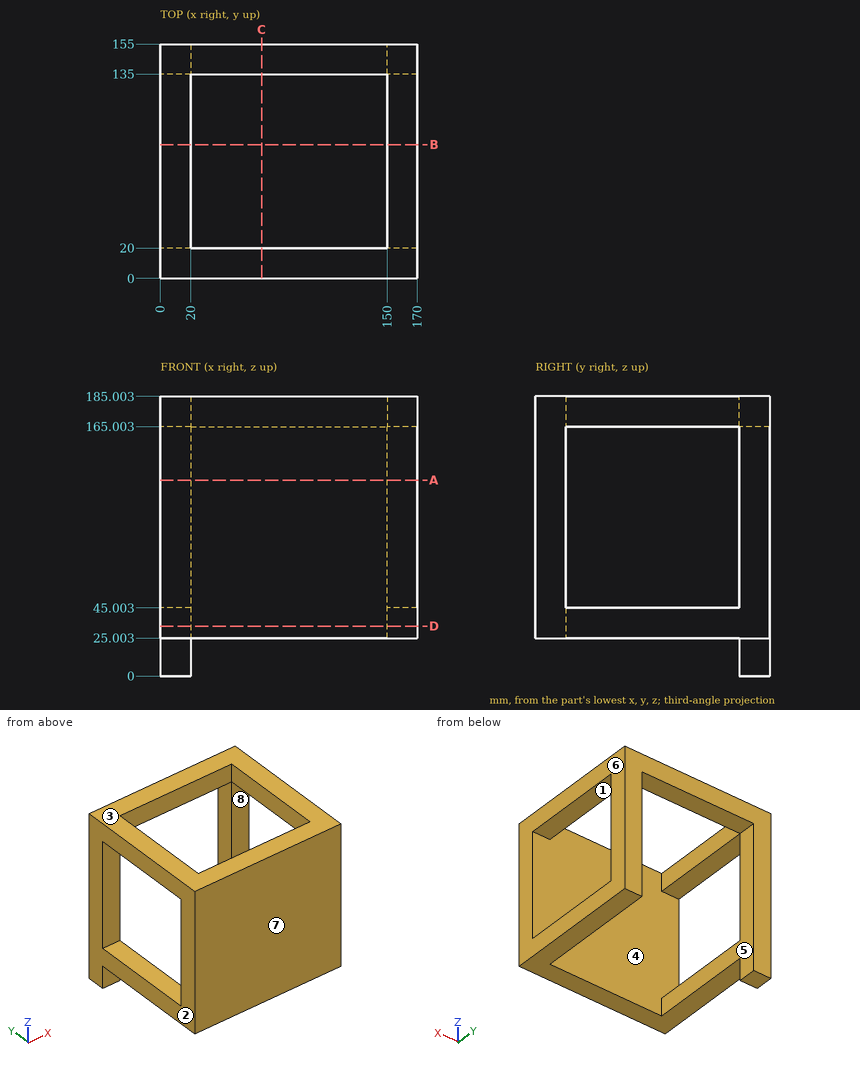
Drawing for the job (mm, zero at the part's lowest x, y, z). A direction names the side the tool comes from. Give positions to 0.01 mm unless a question says otherwise; leave off trailing zeros. Order: outer loops, then holes, each group sorted by start corner. A loop starts at its lowest first (then second) coordinate and runs counter-clockwise, first axis right, second up. Notation, with made-up numbers: M 23,-3 L 53,-3 A25 cw 53,12 Z; hole C 46,73.5 d5. An arc over 180 degrees is marked long. Put each result on its own line as item: value.
Item 1: Probe line 1 (X direction, y = 141, z = 31.5); line 2 (Y direction, x = 7.5, z = 154.5); line 3 (Z direction, x = 153, y = 122). List the from-to ranges inside material, lowest first. Write a range as [from, to].
From the geometry:
line 1: x = [0, 20], [150, 170]
line 2: y = [0, 20], [135, 155]
line 3: z = [25, 45], [165, 185]
Item 2: Slice it at C-C, the plane x = 67. Write the cut outline in (y, z).
From the geometry:
outline: M 0,25 L 20,25 L 20,185 L 0,185 Z; M 135,165 L 155,165 L 155,185 L 135,185 Z
Item 3: Slice it at D-D, the plane z = 33. Write the cut outline in (x, y), plus the area to 3 significant figures.
From the geometry:
outline: M 0,0 L 170,0 L 170,155 L 150,155 L 150,20 L 20,20 L 20,155 L 0,155 Z
area: 8,800 mm2
Item 4: 3-axis set-ups, long thin cutter, end or side, ignore diameter. For the marked faces 4, 5, 6, 7 and 8: which of +Z, -Z, +X, -X, +Y, -Y reach the whole face in a straight line?
From the geometry:
face 4: none
face 5: -Z, +Y
face 6: +Z, -Z, +X, +Y, -Y
face 7: +Z, -Z, +X, -X, -Y
face 8: +X, -X
Item 5: Slice it at B-B, the plane y = 88.5. Write the cut outline in (x, z).
From the geometry:
outline: M 0,25 L 20,25 L 20,45 L 0,45 Z; M 0,165 L 20,165 L 20,185 L 0,185 Z; M 150,25 L 170,25 L 170,45 L 150,45 Z; M 150,165 L 170,165 L 170,185 L 150,185 Z
Item 6: Two-plate mould, pull along Z, no slides. Class the marked faces 1, 2 and 3: +Z half, -Z half, draft (parallel to the pull), parting line (faces both ways), or undercut.
From the geometry:
face 1: undercut
face 2: draft
face 3: +Z half
Item 7: Flat gauge pins, fed straight in: pin 1 Ø6 at (x, z) = (102, 29) entering from -Y; pin 2 Ø16 at (x, y) = (163.5, 104.5) entering from -Z; pin 3 Ø16 at (x, y) = (64.5, 144.5) entering from -Z; pin 4 Ø10 at (x, z) = (8.5, 16) entering from -Y. Where does each tip first touch, or does it go through?
From the geometry:
pin 1: stops at y = 0
pin 2: stops at z = 25
pin 3: stops at z = 165
pin 4: stops at y = 135
Item 8: Slice it at A-A, the plane z = 129.5. Write the cut outline in (x, y), plus the area to 3 significant figures.
From the geometry:
outline: M 0,0 L 170,0 L 170,20 L 0,20 Z; M 0,135 L 20,135 L 20,155 L 0,155 Z; M 150,135 L 170,135 L 170,155 L 150,155 Z
area: 4,200 mm2
